Input: dimensioned drawing with shaded views. Units: mm. Origin: part minimum x, y, z. Coordinates: 2 decimals unless noted, no trailing zeros. Order: outer loops, then holes, each group sorted by start corner. A loop starts at its lowest first (then second) coordinate and runs counter-clockwise, first axis right, second up. Notation, with made-up numbers: (7, 57.5) - (56, 57.5) arc R37 cw to (56, 95.5) - close; hole circle Ø3 at (34, 33.25). An arc over 180 degrees is marked (long way). Use one line per item in the form item = value. Start each with the question number.
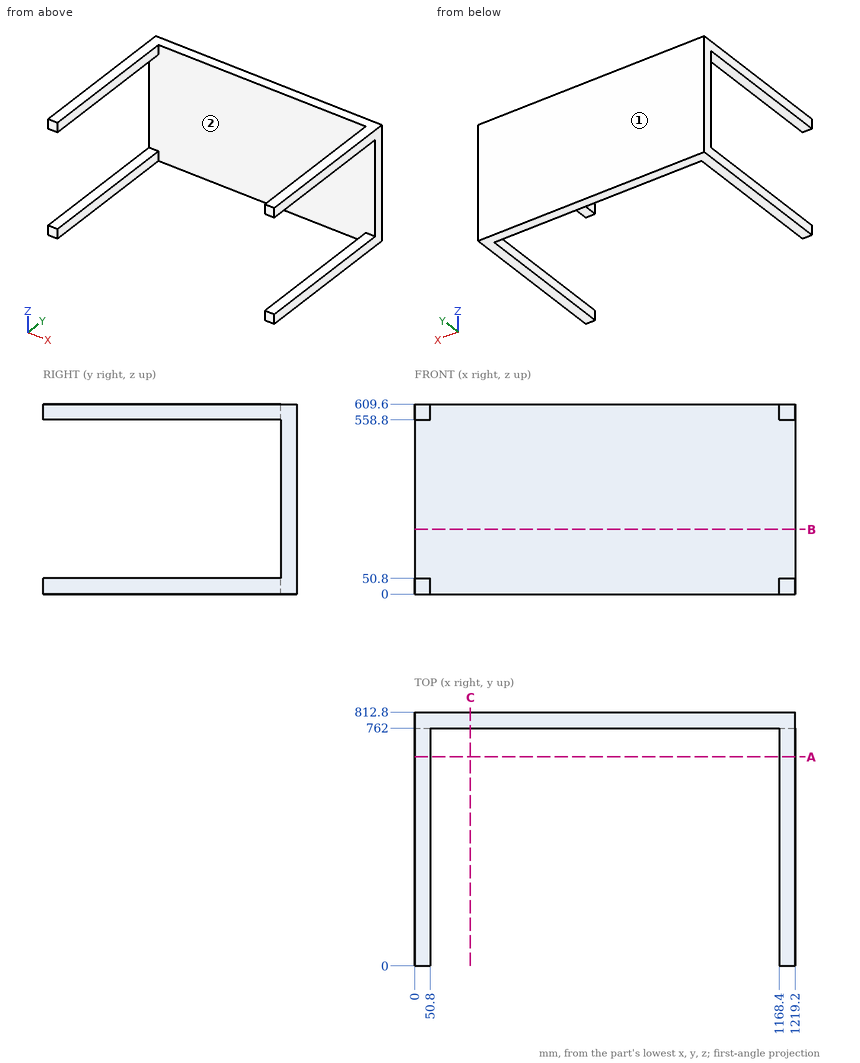
(1) Cut plane A-A on y = 669.5. Return the cut outline in (x, z).
(2) Cut plane B-B on z = 207.5. Return the cut outline in (x, y).
(3) Draft query along X for the marked faces 1 and 2. Return one class per face: released by +X, released by -X, zero draft, split by the parting line, or undercut.
(4) Material intervals for L1, parallel to Z at x = 50.5, y = 735.5; L2, parallel to Y at x = 634.5, z = 126.5; L3, parallel to X at y = 373.5, z = 27, sorted ascending. Write a range as from..to.
(5) Cut plane C-C on x = 178.5. Return the cut outline in (y, z).
Check sheet entries:
q1.outline = (0, 0) - (50.8, 0) - (50.8, 50.8) - (0, 50.8) - close; (0, 558.8) - (50.8, 558.8) - (50.8, 609.6) - (0, 609.6) - close; (1168.4, 0) - (1219.2, 0) - (1219.2, 50.8) - (1168.4, 50.8) - close; (1168.4, 558.8) - (1219.2, 558.8) - (1219.2, 609.6) - (1168.4, 609.6) - close
q2.outline = (0, 762) - (1219.2, 762) - (1219.2, 812.8) - (0, 812.8) - close
q3.face_1 = zero draft
q3.face_2 = undercut
q4.L1 = 0..50.8, 558.8..609.6
q4.L2 = 762..812.8
q4.L3 = 0..50.8, 1168.4..1219.2
q5.outline = (762, 0) - (812.8, 0) - (812.8, 609.6) - (762, 609.6) - close
